```python
from build123d import *

# Parameters (mm, degrees)
SKETCH1_R           = 60
SKETCH1_R_2         = 2.5
BOSS_EXTRUDE1_DEPTH = 15
EXTRUDE_THIN2_DEPTH = 10


with BuildPart() as part:
    # Sketch1 → Boss-Extrude1 (new body)
    with BuildSketch(Plane.XY):
        Circle(SKETCH1_R)
        Circle(SKETCH1_R_2, mode=Mode.SUBTRACT)
    extrude(amount=BOSS_EXTRUDE1_DEPTH)

    # Sketch3 → Extrude-Thin2 (add)
    with BuildSketch(Plane.XY.offset(15)):
        with BuildLine():
            Line((-5.555158991, 58.737894145), (-5.555158991, 78.229038529))
            Line((-5.555158991, 78.229038529), (1, 78.229038529))
            Line((1, 78.229038529), (1, 58.991524815))
            ThreePointArc((1, 58.991524815), (-2.281107294, 58.95588647), (-5.555158991, 58.737894145))
        make_face()
        with BuildLine():
            Line((-4.555158991, 59.826837845), (-4.555158991, 77.229038529))
            Line((-4.555158991, 77.229038529), (0, 77.229038529))
            Line((0, 77.229038529), (0, 60))
            ThreePointArc((0, 60), (-2.27922457, 59.956693833), (-4.555158991, 59.826837845))
        make_face(mode=Mode.SUBTRACT)
        with BuildLine():
            Line((37.60587267, 45.462053855), (51.388193036, 59.244374222))
            Line((51.388193036, 59.244374222), (56.023390411, 54.609176848))
            Line((56.023390411, 54.609176848), (42.42041401, 41.006200448))
            ThreePointArc((42.42041401, 41.006200448), (40.075120678, 43.30109355), (37.60587267, 45.462053855))
        make_face()
        with BuildLine():
            Line((39.082978926, 45.524946549), (51.388193036, 57.83016066))
            Line((51.388193036, 57.83016066), (54.609176848, 54.609176848))
            Line((54.609176848, 54.609176848), (42.426406871, 42.426406871))
            ThreePointArc((42.426406871, 42.426406871), (40.784129637, 44.007439936), (39.082978926, 45.524946549))
        make_face(mode=Mode.SUBTRACT)
        with BuildLine():
            Line((58.737894145, 5.555158991), (78.229038529, 5.555158991))
            Line((78.229038529, 5.555158991), (78.229038529, -1))
            Line((78.229038529, -1), (58.991524815, -1))
            ThreePointArc((58.991524815, -1), (58.95588647, 2.281107294), (58.737894145, 5.555158991))
        make_face()
        with BuildLine():
            Line((59.826837845, 4.555158991), (77.229038529, 4.555158991))
            Line((77.229038529, 4.555158991), (77.229038529, 0))
            Line((77.229038529, 0), (60, 0))
            ThreePointArc((60, 0), (59.956693833, 2.27922457), (59.826837845, 4.555158991))
        make_face(mode=Mode.SUBTRACT)
        with BuildLine():
            Line((45.462053855, -37.60587267), (59.244374222, -51.388193036))
            Line((59.244374222, -51.388193036), (54.609176848, -56.023390411))
            Line((54.609176848, -56.023390411), (41.006200448, -42.42041401))
            ThreePointArc((41.006200448, -42.42041401), (43.30109355, -40.075120678), (45.462053855, -37.60587267))
        make_face()
        with BuildLine():
            Line((45.524946549, -39.082978926), (57.83016066, -51.388193036))
            Line((57.83016066, -51.388193036), (54.609176848, -54.609176848))
            Line((54.609176848, -54.609176848), (42.426406871, -42.426406871))
            ThreePointArc((42.426406871, -42.426406871), (44.007439936, -40.784129637), (45.524946549, -39.082978926))
        make_face(mode=Mode.SUBTRACT)
        with BuildLine():
            Line((5.555158991, -58.737894145), (5.555158991, -78.229038529))
            Line((5.555158991, -78.229038529), (-1, -78.229038529))
            Line((-1, -78.229038529), (-1, -58.991524815))
            ThreePointArc((-1, -58.991524815), (2.281107294, -58.95588647), (5.555158991, -58.737894145))
        make_face()
        with BuildLine():
            Line((4.555158991, -59.826837845), (4.555158991, -77.229038529))
            Line((4.555158991, -77.229038529), (0, -77.229038529))
            Line((0, -77.229038529), (0, -60))
            ThreePointArc((0, -60), (2.27922457, -59.956693833), (4.555158991, -59.826837845))
        make_face(mode=Mode.SUBTRACT)
        with BuildLine():
            Line((-37.60587267, -45.462053855), (-51.388193036, -59.244374222))
            Line((-51.388193036, -59.244374222), (-56.023390411, -54.609176848))
            Line((-56.023390411, -54.609176848), (-42.42041401, -41.006200448))
            ThreePointArc((-42.42041401, -41.006200448), (-40.075120678, -43.30109355), (-37.60587267, -45.462053855))
        make_face()
        with BuildLine():
            Line((-39.082978926, -45.524946549), (-51.388193036, -57.83016066))
            Line((-51.388193036, -57.83016066), (-54.609176848, -54.609176848))
            Line((-54.609176848, -54.609176848), (-42.426406871, -42.426406871))
            ThreePointArc((-42.426406871, -42.426406871), (-40.784129637, -44.007439936), (-39.082978926, -45.524946549))
        make_face(mode=Mode.SUBTRACT)
        with BuildLine():
            Line((-58.737894145, -5.555158991), (-78.229038529, -5.555158991))
            Line((-78.229038529, -5.555158991), (-78.229038529, 1))
            Line((-78.229038529, 1), (-58.991524815, 1))
            ThreePointArc((-58.991524815, 1), (-58.95588647, -2.281107294), (-58.737894145, -5.555158991))
        make_face()
        with BuildLine():
            Line((-59.826837845, -4.555158991), (-77.229038529, -4.555158991))
            Line((-77.229038529, -4.555158991), (-77.229038529, 0))
            Line((-77.229038529, 0), (-60, 0))
            ThreePointArc((-60, 0), (-59.956693833, -2.27922457), (-59.826837845, -4.555158991))
        make_face(mode=Mode.SUBTRACT)
        with BuildLine():
            Line((-45.462053855, 37.60587267), (-59.244374222, 51.388193036))
            Line((-59.244374222, 51.388193036), (-54.609176848, 56.023390411))
            Line((-54.609176848, 56.023390411), (-41.006200448, 42.42041401))
            ThreePointArc((-41.006200448, 42.42041401), (-43.30109355, 40.075120678), (-45.462053855, 37.60587267))
        make_face()
        with BuildLine():
            Line((-45.524946549, 39.082978926), (-57.83016066, 51.388193036))
            Line((-57.83016066, 51.388193036), (-54.609176848, 54.609176848))
            Line((-54.609176848, 54.609176848), (-42.426406871, 42.426406871))
            ThreePointArc((-42.426406871, 42.426406871), (-44.007439936, 40.784129637), (-45.524946549, 39.082978926))
        make_face(mode=Mode.SUBTRACT)
    extrude(amount=-EXTRUDE_THIN2_DEPTH)


solid = part.part
```
Build history of the part. All positions in model axes, mm. A direction names the side the tool comes from. Round coordinates to 2 decimals unless told otherwise and drop trailing zeros. Loops run counter-clockwise (first coordinate to the right, second up) from the corner with the lowest first, then second, coordinate; pieces in that order, holes last.
Item 1: Saw through at C-C (z = 3). List the corners of the cut face in (x, y).
Item 2: Saw through at A-A (x = -64). List the corners of the cut face in (y, z).
Item 3: Which spindle directions (+Z, -Z, +X, -X, +Y, -Y) get a long thin tool onto all of the face, cutting with end or side? Do faces 1 (the face through (52.5, -45.8, 5)), 2 (the face through (-1, -69, 10)), 3 (the face through (-48.252, 49.666, 10.07)), 4 (the face through (-77.229, -2, 10)), 5 (the face through (1, 69, 10)). Say none if no direction does.
Item 4: Drill centre lines: line 1 along Y through (x, z) = (-43.5, 12.25); line 2 along X through (y, z) = (-64, 12.75); line 3 along X through (y, z) = (61.5, 9.5). Where is each one in solid material? Low to high.
Item 5: Saw through at B-B (x = 48). List the corners of the cut face in (y, z).
Item 6: Saw through at D-D (y = -22.5). List the corners of the cut face in (x, z), then the cut area to 3 significant figures.
Item 7: Pin check, flat tips, straight feed: P1, Ø14, axis at x = -43, y = -53, coming from the -Z side; P2, Ø8, axis at x = 40.5, y = -48.5, coming from the -Z side; P3, Ø6, axis at y = 15.5, z = 10.5, coming from the +X side; P4, Ø6, axis at x = -9.5, z = 5, coming from the -Y side. Stop position of each tip, or through.
Worked answers:
1. outline: circle Ø120 at (0, 0); hole circle Ø5 at (0, 0)
2. outline: (-5.56, 5) - (-4.56, 5) - (-4.56, 15) - (-5.56, 15) - close; (0, 5) - (1, 5) - (1, 15) - (0, 15) - close
3. face 1: -Z, +X, -Y
3. face 2: +Z, -Z, -X, -Y
3. face 3: +Z, -Z, +Y
3. face 4: +Z, -Z
3. face 5: +Z, -Z, +X, +Y
4. line 1: y = -51.36 to -49.94, -43.5 to -42.09, -41.32 to 41.32, 43.5 to 44.91
4. line 2: x = -1 to 0, 4.56 to 5.56
4. line 3: x = -5.56 to -4.56, 0 to 1
5. outline: (-49.41, 5) - (-48, 5) - (-48, 15) - (-49.41, 15) - close; (-41.56, 5) - (-40.14, 5) - (-40.14, 15) - (-41.56, 15) - close; (-36, 0) - (36, 0) - (36, 15) - (-36, 15) - close; (46.59, 5) - (48, 5) - (48, 15) - (46.59, 15) - close; (54.44, 5) - (55.86, 5) - (55.86, 15) - (54.44, 15) - close
6. outline: (-55.62, 0) - (55.62, 0) - (55.62, 15) - (-55.62, 15) - close
6. area: 1,670 mm2
7. P1: stops at z = 5
7. P2: stops at z = 0
7. P3: stops at x = 58.68
7. P4: stops at y = -59.65
